from build123d import *

# Parameters (mm, degrees)
F0_R     = 12.5
F0_R_2   = 11.15
F0_R_3   = 6.5
F0_R_4   = 3
F1_DEPTH = 10.25
F2_DEPTH = 8
F3_DEPTH = 15.75


with BuildPart() as f1:
    # F0 (on Top) → F1 (new body, symmetric)
    with BuildSketch(Plane.XY):
        Circle(F0_R)
        Circle(F0_R_2, mode=Mode.SUBTRACT)
        Circle(F0_R_2)
        Circle(F0_R_3, mode=Mode.SUBTRACT)
        Circle(F0_R_3)
        Circle(F0_R_4, mode=Mode.SUBTRACT)
    extrude(amount=F1_DEPTH, both=True)

    # F0 (on Top) → F2 (cut, symmetric)
    with BuildSketch(Plane.XY):
        Circle(F0_R)
        Circle(F0_R_2, mode=Mode.SUBTRACT)
    extrude(amount=F2_DEPTH, both=True, mode=Mode.SUBTRACT)

    # F0 (on Top) → F3 (join)
    with BuildSketch(Plane.XY):
        Circle(F0_R_3)
        Circle(F0_R_4, mode=Mode.SUBTRACT)
    extrude(amount=F3_DEPTH)


solid = f1.part
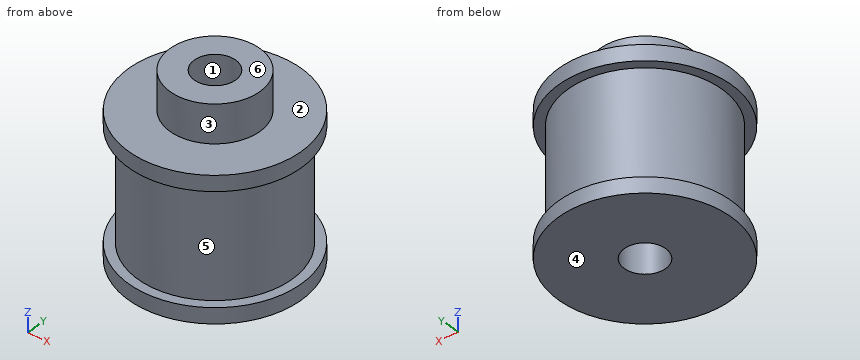
Could you check a few things on this model? Use its own coordinates, in mm. Face numbers are marked on the shaded views. A direction names the side the tool comes from. Coordinates: 2 decimals unless noted, no trailing zeros. Loops run counter-clockwise (first coordinate to the right, second up) from the corner with the lowest first, then second, coordinate; pieces in that order, holes last.
1. Imagine slicing it at C-C (z = 6.75). Please give me the cut outline in (x, y), and give its area (3 significant figures).
2. Imagine slicing it at A-A (y = 0). Please give me the cut outline in (x, z), and give its area (3 significant figures).
3. For P1, Ø3, axis at x = 8, z = -3.5, coming from the +Y side; P2, Ø5, axis at y = 9, z = 7, coming from the -X side; P3, Ø1, axis at y = 4.5, z = 12.5, coming from the -X side; P4, Ø4, axis at x = 0.5, z = 10, coming from the +Y side, each with a flat end and sliding along its axis, tell me the tip position at first contact or that it passes through.
4. I need wall thicknesses on L1, parallel to Y at x = 0, z = 5; L2, parallel to Z at x = 10.25, y = 3.75; L3, parallel to X at y = 8.75, z = 9.5. Which ranges of each line are inside material? Lowest first, please.
5. For the marked faces 1 and 2, which set-ups out of +Z, -Z, +X, -X, +Y, -Y let a thin tool reach every point of the face, with its end or its side?
6. We'd pull the mould along Z, two halves only. Please class the marked faces 3, 4, 5 and 6: released by +Z, released by -Z, zero draft, split by the parting line, or undercut.
7. Imagine slicing it at D-D (x = -6). Please give me the cut outline in (y, z), and give its area (3 significant figures).
Computed values:
1. outline: circle Ø22.3 at (0, 0); hole circle Ø6 at (0, 0)
1. area: 362 mm2
2. outline: (-12.5, -10.25) - (-3, -10.25) - (-3, 15.75) - (-6.5, 15.75) - (-6.5, 10.25) - (-12.5, 10.25) - (-12.5, 8) - (-11.15, 8) - (-11.15, -8) - (-12.5, -8) - close; (3, -10.25) - (12.5, -10.25) - (12.5, -8) - (11.15, -8) - (11.15, 8) - (12.5, 8) - (12.5, 10.25) - (6.5, 10.25) - (6.5, 15.75) - (3, 15.75) - close
2. area: 385 mm2
3. P1: stops at y = 9.06
3. P2: stops at x = -10.55
3. P3: stops at x = -5.12
3. P4: stops at y = 12.5
4. L1: y = -11.15 to -3, 3 to 11.15
4. L2: z = -10.25 to 10.25
4. L3: x = -8.93 to 8.93
5. face 1: +Z, -Z
5. face 2: +Z
6. face 3: zero draft
6. face 4: released by -Z
6. face 5: undercut
6. face 6: released by +Z
7. outline: (-10.97, -10.25) - (10.97, -10.25) - (10.97, -8) - (9.4, -8) - (9.4, 8) - (10.97, 8) - (10.97, 10.25) - (2.5, 10.25) - (2.5, 15.75) - (-2.5, 15.75) - (-2.5, 10.25) - (-10.97, 10.25) - (-10.97, 8) - (-9.4, 8) - (-9.4, -8) - (-10.97, -8) - close
7. area: 427 mm2
